Autodesk Inventor part; units mm, degrees
ref_plane "WorkPlane11" through (0, 0, 0) normal (0, 0, 1) x (1, 0, 0)
ref_plane "Work Plane2" through (0, 0, -4.9) normal (0, 0, 1) x (1, 0, 0)
ref_plane "WorkPlane9" through (0, 0, 8.3) normal (0, 0, 1) x (1, 0, 0)
ref_plane "WorkPlane11" through (0, 0, 0) normal (0, 0, 1) x (1, 0, 0)
ref_plane "Work Plane2" through (0, 0, -4.9) normal (0, 0, 1) x (1, 0, 0)
ref_plane "WorkPlane9" through (0, 0, 8.3) normal (0, 0, 1) x (1, 0, 0)
sketch "Skizze1" plane through (0, 0, 0) normal (0, 0, 1) x (1, 0, 0)
  point P0 (0, 0)
sketch "Skizze2" plane through (0, 0, 0) normal (0, 0, 1) x (1, 0, 0)
  circle A0 centre (0, 0) radius 2.3
  dimension "d2" = 4.6
extrude "Extrusion1" add sketch "Skizze2" against normal blind 0.6
sketch "Skizze3" plane through (0, 0, -0.6) normal (0, 0, -1) x (-1, 0, 0)
  circle A0 centre (0, 0) radius 2.5
  circle A1 centre (0, 0) radius 2.3 construction
  dimension "d8" = 5
extrude "Extrusion2" add sketch "Skizze3" along normal blind 12.7
sketch "Skizze4" plane through (0, 0, 0) normal (0, 0, 1) x (1, 0, 0)
  circle A0 centre (0, 0) radius 4.65
  circle A1 centre (0, 0) radius 2.3 construction
  dimension "d12" = 9.3
extrude "Extrusion3" add sketch "Skizze4" along normal blind 2.7
sketch "Skizze5" plane through (0, 0, 0) normal (0, 1, 0) x (-1, 0, 0)
  line L0 (4.65, 0) -> (2.3, 0)
  line L1 (4.65, 2.35) -> (4.65, 0)
  line L2 (2.3, 0) -> (4.65, 2.35)
  line L3 (-4.65, 0) -> (4.65, 0) construction
  line L4 (0, -7.6493) -> (0, 5.8993)
  line L5 (0, -10.359) -> (0, 8.609)
  line L6 (4.65, 0) -> (4.65, 2.7)
  line L7 (-4.75, 0) -> (4.75, 0)
  line L8 (2.3, 0) -> (2.3, -0.6)
  dimension "d17" = 45
revolve "Drehung1" cut sketch "Skizze5" angle 360 about axis through (0, 0, -7.6493) along (0, 0, 1)
sketch "Skizze6" plane through (0, 0, 0) normal (0, 1, 0) x (-1, 0, 0)
  line L0 (0, 2.7) -> (0, 3.9158)
  line L1 (0, 2.7) -> (4.65, 2.7)
  arc A0 (4.65, 2.7) -> (0, 3.9158) centre (0, -5.5842) ccw
  line L2 (-4.65, 2.7) -> (4.65, 2.7) construction
  line L3 (0, -7.6493) -> (0, 5.8993)
  line L4 (0, -10.359) -> (0, 8.609)
  line L5 (4.65, 2.35) -> (4.65, 2.7)
  arc A1 (0, 3.9158) -> (-4.65, 2.7) centre (0, -5.5842) ccw
  dimension "d20" = 9.5
  dimension "d24" = 4.65
revolve "Drehung2" add sketch "Skizze6" angle 360 about axis through (0, 0, -7.6493) along (0, 0, 1)
fillet "Rundung1" radius 1.3 2 edges at (0, 2.3, 0) (0, -2.3, 0)
chamfer "Fase1" distance 1 distance2 0.2 1 edges at (2.5, 0, -0.6) measured on face at (-2.4919, -0.2012, -9.0667)
sketch "Skizze8" plane through (0, 0, 0) normal (0, 1, 0) x (-1, 0, 0)
  line L0 (-4.65, 3.9158) -> (4.65, 3.9158)
  line L1 (4.65, 3.9158) -> (4.65, 1.9158)
  line L2 (4.65, 1.9158) -> (-4.65, 1.9158)
  line L3 (-4.65, 1.9158) -> (-4.65, 3.9158)
  arc A0 (4.65, 2.7) -> (-4.65, 2.7) centre (0, -5.5842) ccw
  line L4 (-4.65, 2.35) -> (-4.65, 2.7)
  line L5 (4.65, 2.35) -> (4.65, 2.7)
  dimension "msp_d31" = 2
extrude "Extrusion4" cut sketch "Skizze8" against normal mid plane 1.2
thread "Gewinde1"
ref_plane "MSC_PF1" through (0, 0, 0) normal (1, 0, 0) x (0, 1, 0)
ref_plane "MSC_PT1" through (-4.65, 0, 2.35) normal (0, 0, -1) x (-1, 0, 0)
equation "\"d3\" = -msp_x + ParA"
equation "\"d8\" = NND"
equation "\"d9\" = msp_x - ParK + NLG - ParA"
equation "\"d12\" = Dk"
equation "\"d13\" = ParK"
equation "\"d28\" = r"
equation "\"d29\" = msp_x"
equation "\"d30\" = 0.25 * PTC"
equation "\"msp_d31\" = ParT"
equation "\"msp_d32\" = ParN"
equation "\"d2\" = 0.5 * PTC + msp_mdtds"
equation "\"d20\" = rf"
equation "\"d24\" = 0.5 * Dk"
equation "\"PTC\" = 0.8"
equation "\"NND\" = 5"
equation "\"msp_x\" = 1.25 * PTC"
equation "\"NLG\" = 16"
equation "\"msp_mdtds\" = NND - PTC"
equation "\"ParK\" = 2.7"
equation "\"ParN\" = 1.2"
equation "\"ParT\" = 2"
equation "\"r\" = 1.3"
equation "\"prf_c\" = 0"
equation "\"ParA\" = 1.6"
equation "\"Dk\" = 9.3"
equation "\"rf\" = 9.5"
equation "\"ParF\" = 1.2"
equation "\"THREADDIA\" = NND"
equation "\"TEMPLATE\" = 1.2345"
properties part number "DIN EN ISO 2010 - M5x16" material "Messing, weicher Gelbton"
The model under review builds one solid part; all positions refer to its coordinate system, in mm. A direction names the side the tool comes from. Round coordinates to 2 decimals unless told otherwise and drop trailing zeros. Loops run counter-clockwise (first coordinate to the right, second up) from the corner with the lowest first, then second, coordinate; pieces in that order, holes last. Notation, with made-up numbers: (87.25, -34.75) - (97.25, -34.75) arc R13 cw to (97.25, -17.75) - close; hole circle Ø5 at (-34.75, -20.75). An arc over 180 degrees is marked (long way). Write each question's results on one line, items separated by ' | '. Start each with the question number.
Q1. Take a section at A-A on z = -4.75. Give the boundary of the cut face in (x, y), plus the area to 3 significant figures.
Q2. Wall thickness on line 1 along X through (y, z) = (-1.75, -9); line 2 along Z through (x, y) = (3, 2.75); line 3 along Y through (x, z) = (0.75, -10.25): over which ranges is each line inside the solid? List them lowest first. Write a range as [from, to].
Q3. Draft analysis for pull direction Y (two halves, no side actions). For faces 4 (the conical face through (-2.67, -0.84, 0.5)), 5 (the flat face through (0, 0, -13.3)), 6 (the flat face through (0, 0.6, 3)), 7 (the cylindrical face through (-0.09, 4.65, 2.52)), state which applies: pulls with the +Y half, pulls with the -Y half, needs draft (parallel to the pull), parting line crosses it, or undercut.
Q4. Tool access review of faces 1 (the cylindrical face through (0.09, -4.65, 2.52)), 2 (the cylindrical face through (0.54, 2.44, -7.37)), 3 (the flat face through (0, -0.6, 3)): name each direction out of +Z, -Z, +X, -X, +Y, -Y from which nothing blocks a thin tool from reaching the whole face with its end or side.
Q5. Insertion check: P1, Ø5, axis at x = -2, z = -7.5, coming from the +Y side; P2, Ø1.5, axis at x = 2, z = -4.5, coming from the -Y side; P3, Ø0.6, axis at x = 1, y = 0, coming from the +Z side. Each pin has a flat end and moves straight along its axis. Give the tip position at first contact, or say it passes through.
Data:
1) outline: circle Ø5 at (0, 0) | area: 19.6 mm²
2) line 1: x = [-1.79, 1.79] | line 2: z = [1.77, 3] | line 3: y = [-2.38, 2.38]
3) face 4: parting line crosses it | face 5: needs draft | face 6: undercut | face 7: pulls with the +Y half
4) face 1: +Z, -Z, -Y | face 2: -Z | face 3: +Z, +X, -X
5) P1: stops at y = 2.5 | P2: stops at y = -2.17 | P3: stops at z = 1.92
